```python
from build123d import *

# Parameters (mm, degrees)
SKETCH1_W           = 3
SKETCH1_H           = 10
BOSS_EXTRUDE2_DEPTH = 3
SKETCH2_R           = 0.5
CUT_EXTRUDE1_DEPTH  = 132.378270654
FILLET1_R           = 0.5


with BuildPart() as part:
    # Sketch1 → Boss-Extrude2 (new body)
    with BuildSketch(Plane.XY):
        Polygon((-5, 65), (5, 65), (5, 62), (45, 62), (45, 65), (55, 65), (55, 62), (75, 62), (75, 12.5), (81.5, 12.5), (81.5, -12.5), (75, -12.5), (75, -100), (65, -100), (65, -103), (55, -103), (55, -100), (35, -100), (35, -103), (25, -103), (25, -100), (5, -100), (5, -103), (-5, -103), (-5, -100), (-25, -100), (-25, -103), (-35, -103), (-35, -100), (-55, -100), (-55, -103), (-65, -103), (-65, -100), (-75, -100), (-75, -12.5), (-81.5, -12.5), (-81.5, 12.5), (-75, 12.5), (-75, 62), (-55, 62), (-55, 65), (-45, 65), (-45, 62), (-5, 62), align=None)
        with Locations((-73.5, 0)):
            Rectangle(SKETCH1_W, SKETCH1_H, mode=Mode.SUBTRACT)
        with Locations((73.5, 0)):
            Rectangle(SKETCH1_W, SKETCH1_H, mode=Mode.SUBTRACT)
    extrude(amount=BOSS_EXTRUDE2_DEPTH)

    # Sketch2 → Cut-Extrude1 (cut, through all)
    with BuildSketch(Plane.XY.offset(3)):
        with Locations((-72, 5)):
            Circle(SKETCH2_R)
        with Locations((-72, -5)):
            Circle(SKETCH2_R)
        with Locations((-75, 5)):
            Circle(SKETCH2_R)
        with Locations((-75, -5)):
            Circle(SKETCH2_R)
        with Locations((75, -5)):
            Circle(SKETCH2_R)
        with Locations((72, -5)):
            Circle(SKETCH2_R)
        with Locations((72, 5)):
            Circle(SKETCH2_R)
        with Locations((75, 5)):
            Circle(SKETCH2_R)
    extrude(amount=-CUT_EXTRUDE1_DEPTH, mode=Mode.SUBTRACT)

    # Fillet1
    fillet1_edges = [part.edges().sort_by_distance(p)[0] for p in [
        (75, 4.5, 1.5),
        (75, -4.5, 1.5),
        (72.5, -5, 1.5),
        (72, 4.5, 1.5),
        (-72.5, -5, 1.5),
        (-74.5, -5, 1.5),
        (-75, 4.5, 1.5),
        (-72.5, 5, 1.5),
        (74.5, -5, 1.5),
        (-75, -4.5, 1.5),
        (-74.5, 5, 1.5),
        (-72, -4.5, 1.5),
        (72, -4.5, 1.5),
        (72.5, 5, 1.5),
        (74.5, 5, 1.5),
        (-72, 4.5, 1.5),
    ]]
    fillet(fillet1_edges, radius=FILLET1_R)


solid = part.part
```
Can you work these out from the model? Positions are in its coordinate system, mm. Coordinates: 2 decimals unless noted, no trailing zeros. Order: outer loops, then holes, each group sorted by start corner. A loop starts at its lowest first (then second) coordinate and runs counter-clockwise, first axis right, second up.
1. If we section it at A-A (y = -74.5): Please give me the cut outline in (x, z), then the cut area to 3 significant figures.
2. If we section it at C-C (z = 1.3): Give the number of separate pieces and of enclosed holes in the cut face, then the cut area to 3 significant figures.
3. If we section it at B-B (x = -8): Please give me the cut outline in (y, z).
4. I need wall thicknesses on line 1 (X direction, y = 2, z = 0.2); line 2 (Y direction, x = 73.5, z = 2.2); line 3 (X direction, y = -4.5, z = 1.85). Which ranges of each line are inside material? Lowest first, please.
5. I'm going to push flat-ended pins straight in: pin 1 (1.5 mm diameter, centred on x = -43.5, z = 2, fed in from -Y); pin 2 (3 mm diameter, centred on x = 9, y = 17, fed in from -Z); pin 3 (0.9 mm diameter, centred on y = 63, z = 1, fed in from -X); pin 4 (1 mm diameter, centred on x = -73.5, z = 1, fed in from +Y). Where does each tip first touch, or does it pass through?
Entries:
1. outline: (-75, 0) - (75, 0) - (75, 3) - (-75, 3) - close
1. area: 450 mm2
2. separate pieces: 1
2. enclosed holes: 2
2. area: 24,800 mm2
3. outline: (-100, 0) - (62, 0) - (62, 3) - (-100, 3) - close
4. line 1: x = -81.5 to -75, -72 to 72, 75 to 81.5
4. line 2: y = -100 to -5, 5 to 62
4. line 3: x = -81.5 to -75.16, -71.84 to 71.84, 75.16 to 81.5
5. pin 1: stops at y = -100
5. pin 2: stops at z = 0
5. pin 3: stops at x = -55
5. pin 4: stops at y = 62
